Could you check a few things on this model? Use its own coordinates, in mm. Face numbers are marked on the shaded views. A direction names the side the tool comes from. Round coordinates to 2 decimals unless told otherwise and drop trailing zeros. Loops run counter-clockwise (first coordinate to the right, second up) from the corner with the lowest first, then second, coordinate; pieces in that order, holes last. Notation, with made-up numbers: (6.5, 3) -> (65.5, 3) arc R15 cw to (65.5, 14) -> close; hole circle Ø5 at (-37.5, -10.75). An arc over 180 degrees is marked (long way). One line per item, written item: value.
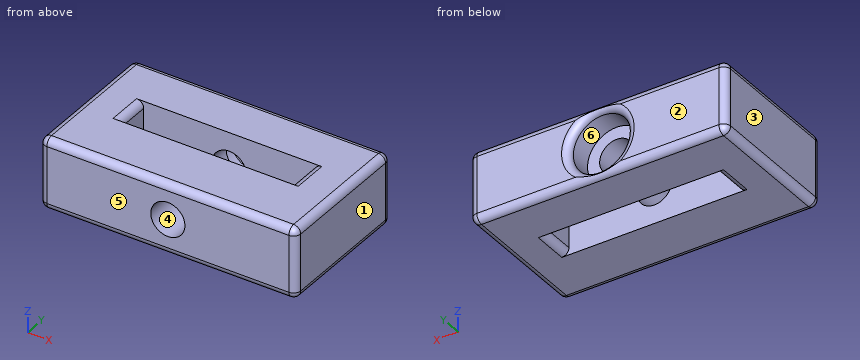
from build123d import *

# Parameters (mm, degrees)
SKETCH1_W           = 12
SKETCH1_H           = 5
BOSS_EXTRUDE1_DEPTH = 4
SKETCH2_W           = 3
SKETCH2_H           = 6.5
BOSS_EXTRUDE2_DEPTH = 5
SKETCH3_W           = 18
SKETCH3_H           = 5
BOSS_EXTRUDE3_DEPTH = 3.5
CUT_EXTRUDE1_REACH  = 15.684
SKETCH4_R           = 1.2
SKETCH5_R           = 2.05
CUT_EXTRUDE2_DEPTH  = 2
FILLET1_R           = 0.5


with BuildPart() as part:
    # Sketch1 → Boss-Extrude1 (new body)
    with BuildSketch(Plane(origin=(0, 0, 0), x_dir=(1, 0, 0), z_dir=(0, 1, 0))):
        Rectangle(SKETCH1_W, SKETCH1_H)
    extrude(amount=BOSS_EXTRUDE1_DEPTH)

    # Sketch2 → Boss-Extrude2 (add)
    with BuildSketch(Plane.XY.offset(2.5)):
        with Locations((-7.5, 3.25)):
            Rectangle(SKETCH2_W, SKETCH2_H)
        with Locations((7.5, 3.25)):
            Rectangle(SKETCH2_W, SKETCH2_H)
    extrude(amount=-BOSS_EXTRUDE2_DEPTH)

    # Sketch3 → Boss-Extrude3 (add)
    with BuildSketch(Plane(origin=(0, 6.5, 0), x_dir=(1, 0, 0), z_dir=(0, 1, 0))):
        Rectangle(SKETCH3_W, SKETCH3_H)
    extrude(amount=BOSS_EXTRUDE3_DEPTH)

    # Cut-Extrude1: up to this face of the body (flat: up to its plane)
    cut_extrude1_end = Plane(part.part.faces().sort_by_distance((0, 0, 0))[0])
    # Sketch4 → Cut-Extrude1 (cut, up to the picked face)
    with BuildSketch(Plane(origin=(0, 10, 0), x_dir=(1, 0, 0), z_dir=(0, 1, 0)), mode=Mode.PRIVATE) as cut_extrude1_sk1:
        with Locations(Location((0, 0, 0), (0, 0, 270))):
            Circle(SKETCH4_R)
    cut_extrude1_tool1 = split(extrude(cut_extrude1_sk1.sketch, amount=-CUT_EXTRUDE1_REACH, mode=Mode.PRIVATE), bisect_by=cut_extrude1_end, keep=Keep.BOTH, mode=Mode.PRIVATE)
    add(cut_extrude1_tool1.solids().sort_by(Axis((0, 10, 0), (0, -1, 0)))[0], mode=Mode.SUBTRACT)

    # Sketch5 → Cut-Extrude2 (cut)
    with BuildSketch(Plane(origin=(0, 10, 0), x_dir=(1, 0, 0), z_dir=(0, 1, 0))):
        with Locations(Location((0, 0, 0), (0, 0, 270))):
            Circle(SKETCH5_R)
    extrude(amount=-CUT_EXTRUDE2_DEPTH, mode=Mode.SUBTRACT)

    # Fillet1
    # the kernel refuses this fillet: 0.5 mm, written as the material it takes off along each edge
    with BuildSketch(Plane(origin=(-8.5, 0.5, 2), x_dir=(0, -1, 0), z_dir=(0, 0, 1))) as fillet1_piece_1_section:
        Polygon((0, 0), (FILLET1_R, 0), (FILLET1_R, -FILLET1_R), (0, -FILLET1_R), align=None)
    fillet1_piece_1 = extrude(amount=FILLET1_R, mode=Mode.PRIVATE)
    fillet1_piece_1 = fillet1_piece_1 - Plane(origin=(-8.5, 0.5, 2), x_dir=(0.7071067811865475, 0.7071067811865475, 0), z_dir=(0, 0, 1)) * Sphere(FILLET1_R, mode=Mode.PRIVATE)
    add(fillet1_piece_1, mode=Mode.SUBTRACT)
    with BuildSketch(Plane(origin=(-8.5, 0.5, -2), x_dir=(-1, 0, 0), z_dir=(0, -1, 0))) as fillet1_piece_2_section:
        Polygon((0, 0), (FILLET1_R, 0), (FILLET1_R, FILLET1_R), (0, FILLET1_R), align=None)
    fillet1_piece_2 = extrude(amount=FILLET1_R, mode=Mode.PRIVATE)
    fillet1_piece_2 = fillet1_piece_2 - Plane(origin=(-8.5, 0.5, -2), x_dir=(0.7071067811865475, 0, 0.7071067811865475), z_dir=(0, -1, 0)) * Sphere(FILLET1_R, mode=Mode.PRIVATE)
    add(fillet1_piece_2, mode=Mode.SUBTRACT)
    with BuildSketch(Plane(origin=(-8.5, 9.5, 2), x_dir=(-1, 0, 0), z_dir=(0, 0, 1))) as fillet1_piece_3_section:
        Polygon((0, 0), (FILLET1_R, 0), (FILLET1_R, -FILLET1_R), (0, -FILLET1_R), align=None)
    fillet1_piece_3 = extrude(amount=FILLET1_R, mode=Mode.PRIVATE)
    fillet1_piece_3 = fillet1_piece_3 - Plane(origin=(-8.5, 9.5, 2), x_dir=(0.7071067811865475, -0.7071067811865475, 0), z_dir=(0, 0, 1)) * Sphere(FILLET1_R, mode=Mode.PRIVATE)
    add(fillet1_piece_3, mode=Mode.SUBTRACT)
    with BuildSketch(Plane(origin=(-8.5, 9.5, -2), x_dir=(-1, 0, 0), z_dir=(0, 0, -1))) as fillet1_piece_4_section:
        Polygon((0, 0), (FILLET1_R, 0), (FILLET1_R, FILLET1_R), (0, FILLET1_R), align=None)
    fillet1_piece_4 = extrude(amount=FILLET1_R, mode=Mode.PRIVATE)
    fillet1_piece_4 = fillet1_piece_4 - Plane(origin=(-8.5, 9.5, -2), x_dir=(0.7071067811865475, -0.7071067811865475, 0), z_dir=(0, 0, -1)) * Sphere(FILLET1_R, mode=Mode.PRIVATE)
    add(fillet1_piece_4, mode=Mode.SUBTRACT)
    with BuildSketch(Plane(origin=(8.5, 0.5, 2), x_dir=(0, -1, 0), z_dir=(0, 0, 1))) as fillet1_piece_5_section:
        Polygon((0, 0), (FILLET1_R, 0), (FILLET1_R, FILLET1_R), (0, FILLET1_R), align=None)
    fillet1_piece_5 = extrude(amount=FILLET1_R, mode=Mode.PRIVATE)
    fillet1_piece_5 = fillet1_piece_5 - Plane(origin=(8.5, 0.5, 2), x_dir=(-0.7071067811865476, 0.7071067811865475, 0), z_dir=(0, 0, 1)) * Sphere(FILLET1_R, mode=Mode.PRIVATE)
    add(fillet1_piece_5, mode=Mode.SUBTRACT)
    with BuildSketch(Plane(origin=(8.5, 0.5, -2), x_dir=(1, 0, 0), z_dir=(0, -1, 0))) as fillet1_piece_6_section:
        Polygon((0, 0), (FILLET1_R, 0), (FILLET1_R, -FILLET1_R), (0, -FILLET1_R), align=None)
    fillet1_piece_6 = extrude(amount=FILLET1_R, mode=Mode.PRIVATE)
    fillet1_piece_6 = fillet1_piece_6 - Plane(origin=(8.5, 0.5, -2), x_dir=(-0.7071067811865475, 0, 0.7071067811865475), z_dir=(0, -1, 0)) * Sphere(FILLET1_R, mode=Mode.PRIVATE)
    add(fillet1_piece_6, mode=Mode.SUBTRACT)
    with BuildSketch(Plane(origin=(8.5, 9.5, 2), x_dir=(0, 1, 0), z_dir=(0, 0, 1))) as fillet1_piece_7_section:
        Polygon((0, 0), (FILLET1_R, 0), (FILLET1_R, -FILLET1_R), (0, -FILLET1_R), align=None)
    fillet1_piece_7 = extrude(amount=FILLET1_R, mode=Mode.PRIVATE)
    fillet1_piece_7 = fillet1_piece_7 - Plane(origin=(8.5, 9.5, 2), x_dir=(-0.7071067811865475, -0.7071067811865477, 0), z_dir=(0, 0, 1)) * Sphere(FILLET1_R, mode=Mode.PRIVATE)
    add(fillet1_piece_7, mode=Mode.SUBTRACT)
    with BuildSketch(Plane(origin=(8.5, 9.5, -2), x_dir=(0, 1, 0), z_dir=(0, 0, -1))) as fillet1_piece_8_section:
        Polygon((0, 0), (FILLET1_R, 0), (FILLET1_R, FILLET1_R), (0, FILLET1_R), align=None)
    fillet1_piece_8 = extrude(amount=FILLET1_R, mode=Mode.PRIVATE)
    fillet1_piece_8 = fillet1_piece_8 - Plane(origin=(8.5, 9.5, -2), x_dir=(-0.7071067811865475, -0.7071067811865477, 0), z_dir=(0, 0, -1)) * Sphere(FILLET1_R, mode=Mode.PRIVATE)
    add(fillet1_piece_8, mode=Mode.SUBTRACT)
    with BuildSketch(Plane(origin=(-9, 0, 2), x_dir=(1, 0, 0), z_dir=(0, 0, -1)), Plane(origin=(-9, 10, 2), x_dir=(0, -1, 0), z_dir=(0, 0, -1))) as fillet1_piece_9:
        with BuildLine():
            CenterArc((FILLET1_R, -FILLET1_R), FILLET1_R, 90, 90)
            Line((0, -FILLET1_R), (0, 0))
            Line((0, 0), (FILLET1_R, 0))
        make_face()
    extrude(amount=4, mode=Mode.SUBTRACT)
    with BuildSketch(Plane(origin=(-6, 4, 2.5), x_dir=(-1, 0, 0), z_dir=(0, 1, 0)), Plane(origin=(-6, 4, -2.5), x_dir=(0, 0, 1), z_dir=(0, 1, 0))) as fillet1_piece_10:
        with BuildLine():
            CenterArc((FILLET1_R, -FILLET1_R), FILLET1_R, 90, 90)
            Line((0, -FILLET1_R), (0, 0))
            Line((0, 0), (FILLET1_R, 0))
        make_face()
    extrude(amount=2.5, mode=Mode.SUBTRACT)
    with BuildSketch(Plane(origin=(-9, 9.5, 2.5), x_dir=(1, 0, 0), z_dir=(0, -1, 0)), Plane(origin=(-9, 9.5, -2.5), x_dir=(0, 0, 1), z_dir=(0, -1, 0)), Plane(origin=(9, 0.5, 2.5), x_dir=(-1, 0, 0), z_dir=(0, 1, 0)), Plane(origin=(9, 0.5, -2.5), x_dir=(0, 0, 1), z_dir=(0, 1, 0))) as fillet1_piece_11:
        with BuildLine():
            CenterArc((FILLET1_R, -FILLET1_R), FILLET1_R, 90, 90)
            Line((0, -FILLET1_R), (0, 0))
            Line((0, 0), (FILLET1_R, 0))
        make_face()
    extrude(amount=9, mode=Mode.SUBTRACT)
    with BuildSketch(Plane(origin=(9, 0, 2), x_dir=(-1, 0, 0), z_dir=(0, 0, -1)), Plane(origin=(9, 10, -2), x_dir=(-1, 0, 0), z_dir=(0, 0, 1))) as fillet1_piece_12:
        with BuildLine():
            CenterArc((FILLET1_R, FILLET1_R), FILLET1_R, 180, 90)
            Line((0, FILLET1_R), (0, 0))
            Line((0, 0), (FILLET1_R, 0))
        make_face()
    extrude(amount=4, mode=Mode.SUBTRACT)
    with BuildSketch(Plane(origin=(6, 4, 2.5), x_dir=(1, 0, 0), z_dir=(0, 1, 0)), Plane(origin=(6, 4, -2.5), x_dir=(0, 0, 1), z_dir=(0, 1, 0))) as fillet1_piece_13:
        with BuildLine():
            CenterArc((FILLET1_R, FILLET1_R), FILLET1_R, 180, 90)
            Line((0, FILLET1_R), (0, 0))
            Line((0, 0), (FILLET1_R, 0))
        make_face()
    extrude(amount=2.5, mode=Mode.SUBTRACT)
    with BuildSketch(Plane(origin=(8.5, 10, 2.5), x_dir=(0, -1, 0), z_dir=(-1, 0, 0)), Plane(origin=(-8.5, 0, 2.5), x_dir=(0, 1, 0), z_dir=(1, 0, 0)), Plane(origin=(-8.5, 0, -2.5), x_dir=(0, 0, 1), z_dir=(1, 0, 0))) as fillet1_piece_14:
        with BuildLine():
            CenterArc((FILLET1_R, -FILLET1_R), FILLET1_R, 90, 90)
            Line((0, -FILLET1_R), (0, 0))
            Line((0, 0), (FILLET1_R, 0))
        make_face()
    extrude(amount=17, mode=Mode.SUBTRACT)
    with BuildSketch(Plane(origin=(-8.5, 10, -2.5), x_dir=(0, 0, 1), z_dir=(1, 0, 0))) as fillet1_piece_15:
        with BuildLine():
            CenterArc((FILLET1_R, FILLET1_R), FILLET1_R, 180, 90)
            Line((0, FILLET1_R), (0, 0))
            Line((0, 0), (FILLET1_R, 0))
        make_face()
    extrude(amount=17, mode=Mode.SUBTRACT)
    with BuildSketch(Plane(origin=(0, 10, 0), x_dir=(0, 0, 1), z_dir=(-1, 0, 0))) as fillet1_piece_16:
        with BuildLine():
            CenterArc((2.05 + FILLET1_R, -FILLET1_R), FILLET1_R, 90, 90)
            Line((2.05, -FILLET1_R), (2.05, 0))
            Line((2.05, 0), (2.05 + FILLET1_R, 0))
        make_face()
    revolve(axis=Axis((0, 10, 0), (0, 1, 0)), mode=Mode.SUBTRACT)


solid = part.part
(1) If we section it at A-A, the plane x = -4.5: Please give me the cut outline in (y, z), then the cut area to 3 significant figures.
Recorded:
outline: (0, -2) arc R0.5 ccw to (0.5, -2.5) -> (4, -2.5) -> (4, 2.5) -> (0.5, 2.5) arc R0.5 ccw to (0, 2) -> close; (6.5, -2.5) -> (9.5, -2.5) arc R0.5 ccw to (10, -2) -> (10, 2) arc R0.5 ccw to (9.5, 2.5) -> (6.5, 2.5) -> close
area: 37.3 mm²
(2) If we section it at B-B, the plane z = 0: Please give me the cut outline in (x, y).
Recorded:
outline: (-9, 0.5) arc R0.5 ccw to (-8.5, 0) -> (-1.2, 0) -> (-1.2, 4) -> (-6, 4) -> (-6, 6.5) -> (-1.2, 6.5) -> (-1.2, 8) -> (-2.05, 8) -> (-2.05, 9.5) arc R0.5 ccw to (-2.55, 10) -> (-8.5, 10) arc R0.5 ccw to (-9, 9.5) -> close; (1.2, 0) -> (8.5, 0) arc R0.5 ccw to (9, 0.5) -> (9, 9.5) arc R0.5 ccw to (8.5, 10) -> (2.55, 10) arc R0.5 ccw to (2.05, 9.5) -> (2.05, 8) -> (1.2, 8) -> (1.2, 6.5) -> (6, 6.5) -> (6, 4) -> (1.2, 4) -> close
(3) If I drill on L1, parallel to Y at x = 0.25, z = 1.8; L2, parallel to X at y = 7.35, z = 0; L3, parallel to Y at x = -4.75, z = -0.8, over which ranges is the centre line in solid material (lowest first)?
Recorded:
L1: 0 to 4, 6.5 to 8
L2: -9 to -1.2, 1.2 to 9
L3: 0 to 4, 6.5 to 10
(4) If we section it at D-D, the plane y = 6: Please give me the cut outline in (x, z), then the cut area to 3 significant figures.
Recorded:
outline: (-9, -2) arc R0.5 ccw to (-8.5, -2.5) -> (-6.5, -2.5) arc R0.5 ccw to (-6, -2) -> (-6, 2) arc R0.5 ccw to (-6.5, 2.5) -> (-8.5, 2.5) arc R0.5 ccw to (-9, 2) -> close; (6, -2) arc R0.5 ccw to (6.5, -2.5) -> (8.5, -2.5) arc R0.5 ccw to (9, -2) -> (9, 2) arc R0.5 ccw to (8.5, 2.5) -> (6.5, 2.5) arc R0.5 ccw to (6, 2) -> close
area: 29.6 mm²
(5) I'm going to push flat-ended pins straight in: pin 1 Ø2 at (x, z) = (0, 0) entering from +Y; pin 2 Ø2 at (x, z) = (0, -1) entering from +Y. Where does each tip first touch, or does it pass through?
Recorded:
pin 1: through
pin 2: y = 8
(6) Thinking about a two-plate mould opening in X: for the marked faces 1, 2, 3 and 4, which applies, released by +X, released by -X, zero draft, split by the parting line, or undercut?
Recorded:
face 1: released by +X
face 2: zero draft
face 3: released by -X
face 4: undercut
(7) If we section it at C-C, the plane y = 1: Please give me the cut outline in (x, z).
Recorded:
outline: (-9, -2) arc R0.5 ccw to (-8.5, -2.5) -> (8.5, -2.5) arc R0.5 ccw to (9, -2) -> (9, 2) arc R0.5 ccw to (8.5, 2.5) -> (-8.5, 2.5) arc R0.5 ccw to (-9, 2) -> close; hole circle Ø2.4 at (0, 0)
(8) For the marked faces 5 and 6, which set-ups out of +Z, -Z, +X, -X, +Y, -Y let a thin tool reach every point of the face, with its end or its side?
Recorded:
face 5: +Z, -Z, +X, -X, -Y
face 6: +Y
